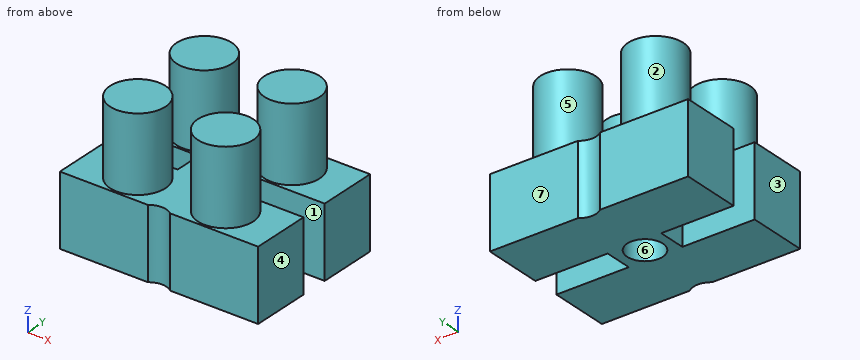
```python
from build123d import *

# Parameters (mm, degrees)
SKETCH1_W                 = 18.2372
SKETCH1_H                 = 13.4874
BOSS_EXTRUDE1_DEPTH       = 6.5024
SKETCH2_W                 = 6.6548
SKETCH2_H                 = 2.54
CUT_EXTRUDE1_DEPTH        = 14.073161875
SKETCH5_R                 = 2.54
BOSS_EXTRUDE2_DEPTH       = 6.858
SKETCH6_W                 = 18.2372
SKETCH6_H                 = 5.4737
CUT_EXTRUDE2_DEPTH        = 14.253622888
F_4_CLEARANCE_HOLE1_D     = 3.2639
LPATTERN1_COUNT           = 4
LPATTERN1_PITCH           = 8.001
LPATTERN1_COPY_1_SKETCH_W = 6.6548
LPATTERN1_COPY_1_SKETCH_H = 2.54
LPATTERN1_COPY_1_DEPTH    = 14.073161875
LPATTERN1_COPY_2_SKETCH_W = 6.6548
LPATTERN1_COPY_2_SKETCH_H = 2.54
LPATTERN1_COPY_2_DEPTH    = 14.073161875
LPATTERN1_COPY_3_SKETCH_W = 6.6548
LPATTERN1_COPY_3_SKETCH_H = 2.54
LPATTERN1_COPY_3_DEPTH    = 14.073161875
LPATTERN1_COPY_4_SKETCH_R = 2.54
LPATTERN1_COPY_4_DEPTH    = 6.858
LPATTERN1_COPY_5_SKETCH_R = 2.54
LPATTERN1_COPY_5_DEPTH    = 6.858
LPATTERN1_COPY_6_SKETCH_R = 2.54
LPATTERN1_COPY_6_DEPTH    = 6.858
SKETCH7_W                 = 18.2372
SKETCH7_H                 = 8.0137
CUT_EXTRUDE3_DEPTH        = 33.795435519
SKETCH8_W                 = 18.2372
SKETCH8_H                 = 16.0147
CUT_EXTRUDE5_DEPTH        = 28.900509729


with BuildPart() as part:
    # Sketch1 → Boss-Extrude1 (new body)
    with BuildSketch(Plane.XY):
        Rectangle(SKETCH1_W, SKETCH1_H)
    boss_extrude1 = extrude(amount=BOSS_EXTRUDE1_DEPTH)

    # Sketch2 → Cut-Extrude1 (cut, through all)
    with BuildSketch(Plane.XY.offset(6.5024)):
        with Locations((5.7912, 0)):
            Rectangle(SKETCH2_W, SKETCH2_H)
    cut_extrude1 = extrude(amount=-CUT_EXTRUDE1_DEPTH, mode=Mode.SUBTRACT)

    # Sketch5 → Boss-Extrude2 (add)
    with BuildSketch(Plane.XY.offset(6.5024)):
        with Locations(Location((4.0386, -4.00685, 0), (0, 0, 180))):
            Circle(SKETCH5_R)
    boss_extrude2 = extrude(amount=BOSS_EXTRUDE2_DEPTH)

    # Sketch6 → Cut-Extrude2 (cut, through all)
    with BuildSketch(Plane.XY.offset(6.5024)):
        with Locations((0, 4.00685)):
            Rectangle(SKETCH6_W, SKETCH6_H)
    extrude(amount=-CUT_EXTRUDE2_DEPTH, mode=Mode.SUBTRACT)

    # #4 Clearance Hole1 (through all)
    with Locations(Plane.XY.offset(6.5024)):
        with Locations((0, 0)):
            f_4_clearance_hole1 = Hole(F_4_CLEARANCE_HOLE1_D / 2)

    # Mirror4: Cut-Extrude1, Boss-Extrude2 across plane
    add(cut_extrude1.mirror(Plane(origin=(0, 0, 0), x_dir=(0, 0, 1), z_dir=(1, 0, 0))), mode=Mode.SUBTRACT)
    add(boss_extrude2.mirror(Plane(origin=(0, 0, 0), x_dir=(0, 0, 1), z_dir=(1, 0, 0))))

    # LPattern1: Boss-Extrude1, Cut-Extrude1, Boss-Extrude2, #4 Clearance Hole1 ×4
    with Locations(*[(0, i * LPATTERN1_PITCH, 0) for i in range(1, LPATTERN1_COUNT)]):
        add(boss_extrude1)
        add(cut_extrude1, mode=Mode.SUBTRACT)
        add(boss_extrude2)
        add(f_4_clearance_hole1, mode=Mode.SUBTRACT)

    # LPattern1 copy 1 sketch → LPattern1 copy 1 (cut, through all)
    with BuildSketch(Plane(origin=(0, 8.001, 6.5024), x_dir=(-1, 0, 0), z_dir=(0, 0, 1))):
        with Locations((5.7912, 0)):
            Rectangle(LPATTERN1_COPY_1_SKETCH_W, LPATTERN1_COPY_1_SKETCH_H)
    extrude(amount=-LPATTERN1_COPY_1_DEPTH, mode=Mode.SUBTRACT)

    # LPattern1 copy 2 sketch → LPattern1 copy 2 (cut, through all)
    with BuildSketch(Plane(origin=(0, 16.002, 6.5024), x_dir=(-1, 0, 0), z_dir=(0, 0, 1))):
        with Locations((5.7912, 0)):
            Rectangle(LPATTERN1_COPY_2_SKETCH_W, LPATTERN1_COPY_2_SKETCH_H)
    extrude(amount=-LPATTERN1_COPY_2_DEPTH, mode=Mode.SUBTRACT)

    # LPattern1 copy 3 sketch → LPattern1 copy 3 (cut, through all)
    with BuildSketch(Plane(origin=(0, 24.003, 6.5024), x_dir=(-1, 0, 0), z_dir=(0, 0, 1))):
        with Locations((5.7912, 0)):
            Rectangle(LPATTERN1_COPY_3_SKETCH_W, LPATTERN1_COPY_3_SKETCH_H)
    extrude(amount=-LPATTERN1_COPY_3_DEPTH, mode=Mode.SUBTRACT)

    # LPattern1 copy 4 sketch → LPattern1 copy 4 (add)
    with BuildSketch(Plane(origin=(0, 8.001, 6.5024), x_dir=(-1, 0, 0), z_dir=(0, 0, 1))):
        with Locations((4.0386, 4.00685)):
            Circle(LPATTERN1_COPY_4_SKETCH_R)
    extrude(amount=LPATTERN1_COPY_4_DEPTH)

    # LPattern1 copy 5 sketch → LPattern1 copy 5 (add)
    with BuildSketch(Plane(origin=(0, 16.002, 6.5024), x_dir=(-1, 0, 0), z_dir=(0, 0, 1))):
        with Locations((4.0386, 4.00685)):
            Circle(LPATTERN1_COPY_5_SKETCH_R)
    extrude(amount=LPATTERN1_COPY_5_DEPTH)

    # LPattern1 copy 6 sketch → LPattern1 copy 6 (add)
    with BuildSketch(Plane(origin=(0, 24.003, 6.5024), x_dir=(-1, 0, 0), z_dir=(0, 0, 1))):
        with Locations((4.0386, 4.00685)):
            Circle(LPATTERN1_COPY_6_SKETCH_R)
    extrude(amount=LPATTERN1_COPY_6_DEPTH)

    # Sketch7 → Cut-Extrude3 (cut, through all)
    with BuildSketch(Plane.XY.offset(6.5024)):
        with Locations((0, 26.73985)):
            Rectangle(SKETCH7_W, SKETCH7_H)
    extrude(amount=-CUT_EXTRUDE3_DEPTH, mode=Mode.SUBTRACT)

    # Sketch8 → Cut-Extrude5 (cut, through all)
    with BuildSketch(Plane.XY):
        with Locations((0, 1.26365)):
            Rectangle(SKETCH8_W, SKETCH8_H)
    extrude(amount=CUT_EXTRUDE5_DEPTH, mode=Mode.SUBTRACT)


solid = part.part
```
Model file for the job. Use its own axes, mm. Face numbers are marked on the shaded views. A direction names the side the tool comes from. Round coordinates to 2 decimals unless told otherwise and drop trailing zeros. Order: outer loops, then holes, each group sorted by start corner. A loop starts at its lowest first (then second) coordinate and runs counter-clockwise, first axis right, second up. Notation, with made-up numbers: (2.25, -32) -> (21.25, -32) arc R27 cw to (21.25, 6) -> close; hole circle Ø8 at (50.25, -19.75). An arc over 180 degrees is marked (long way). Use one line per item in the form item = value.
Item 1: Flat gauge pins, fed straight in: pin 1 Ø2 at (y, z) = (20.5, 9) entering from -X; pin 2 Ø2.5 at (x, y) = (0, 16.002) entering from -Z; pin 3 Ø1.3 at (y, z) = (16.5, 2) entering from -X. Where does each tip first touch, or does it go through?
Returned:
pin_1 = -6.58
pin_2 = through
pin_3 = -2.46
Item 2: Cut at B-B, the plane z = 1.5. Write the cut outline in (x, y), and give its area (3 significant figures).
Returned:
outline = (-9.12, 9.27) -> (-1.02, 9.27) arc R1.63 cw to (1.02, 9.27) -> (9.12, 9.27) -> (9.12, 14.73) -> (2.46, 14.73) -> (2.46, 17.27) -> (9.12, 17.27) -> (9.12, 22.73) -> (1.02, 22.73) arc R1.63 cw to (-1.02, 22.73) -> (-9.12, 22.73) -> (-9.12, 17.27) -> (-2.46, 17.27) -> (-2.46, 14.73) -> (-9.12, 14.73) -> close; hole circle Ø3.26 at (0, 16)
area = 202 mm^2
Item 3: Drill centre lines: line 1 (Y direction, x = -5.5, z = 3.25); line 2 (Y direction, x = -4, z = 9.25); line 3 (Z direction, x = -1.25, y = 18.5). Where is each one in solid material? Low to high.
Returned:
line_1 = 9.27 to 14.73, 17.27 to 22.73
line_2 = 9.46 to 14.53, 17.46 to 22.54
line_3 = 0 to 6.5
Item 4: Pull direction X, two halves, no side cores. Call the marked faces 4, 5, 6 and 7: released by +X, released by -X, zero draft, split by the parting line, or undercut.
Returned:
face_4 = released by +X
face_5 = undercut
face_6 = undercut
face_7 = zero draft
Item 5: Cut at A-A, the plane x = 7.5. Write the cut outline in (y, z).
Returned:
outline = (9.27, 0) -> (14.73, 0) -> (14.73, 6.5) -> (9.27, 6.5) -> close; (17.27, 0) -> (22.73, 0) -> (22.73, 6.5) -> (17.27, 6.5) -> close
Item 6: Tool access for the marked faces 1, 2 and 3: list every direction of +Z, -Z, +X, -X, +Y, -Y with a clear straight run to the whole face (end or side of a thin tool).
Returned:
face_1 = +Z, -Z, +X
face_2 = +Z
face_3 = +Z, -Z, -X, +Y, -Y
Item 7: Cut at D-D, the plane x = 0. Write the cut outline in (y, z), and give its area (3 significant figures).
Returned:
outline = (9.63, 0) -> (14.37, 0) -> (14.37, 6.5) -> (9.63, 6.5) -> close; (17.63, 0) -> (22.37, 0) -> (22.37, 6.5) -> (17.63, 6.5) -> close
area = 61.6 mm^2
Item 8: Cut at C-C, the plane y = 19.75. Write the cut outline in (x, z), and give its area (3 significant figures).
Returned:
outline = (-9.12, 0) -> (9.12, 0) -> (9.12, 6.5) -> (6.57, 6.5) -> (6.57, 13.36) -> (1.51, 13.36) -> (1.51, 6.5) -> (-1.51, 6.5) -> (-1.51, 13.36) -> (-6.57, 13.36) -> (-6.57, 6.5) -> (-9.12, 6.5) -> close
area = 188 mm^2
